Input: part model. Units: mm. Frame: model coordinates. Give positions to 0.01 mm unless a question says otherwise; leave off trailing zeros. Write each loop counter-clockwise with the first axis right and the second up, starting at its lowest first coordinate (ties: lowest second). Pieces come first, ordered by that corner, then holes. Notation, with made-up numbers: (-19.5, 11) - (33.5, 11) arc R19 cw to (33.5, 35) - close; hole circle Ø10 at (75.5, 37.5). An arc over 180 degrees is marked (long way). Use a Markdown table: item, result. Add a question column.
1. Section query C-C, the plane x = 3.55. Return loops of the section in (y, z), plus the area to 3 significant figures.
2. Section query D-D, the plane z = -0.25. Return loops of the section in (x, y), plus the area to 3 significant figures.
3. Section query B-B, the plane z = 5. Return loops of the section in (x, y), plus the area to 3 significant figures.
4. Mould query, pull axis Z, two halves, no side actions, for faces 1 (the cylindrical face through (1.87, 1.58, 5.76)), 2 (the flat face through (3, 2, -7.46)), 3 (the flat face through (4, 3.2, 0)). Classes: released by +Z, released by -Z, zero draft, split by the parting line, or undercut.
5. Material intervals for probe 1 along Z at (x, y) = (2.8, 2); probe 2 along X at (y, z) = (1.75, 5); probe 3 along Z at (x, y) = (3.2, 0.45), sorted ascending.
6. Section query A-A, the plane y = 2.5. Return loops of the section in (x, z).
```python
from build123d import *

# Parameters (mm, degrees)
SKETCH1_W           = 5.409
SKETCH1_H           = 3.2004
BOSS_EXTRUDE1_DEPTH = 7.459999939
SKETCH3_R           = 1.1303
CUT_EXTRUDE1_DEPTH  = 3.2004
FILLET1_R           = 0.762


with BuildPart() as part:
    # Sketch1 → Boss-Extrude1 (new body, symmetric)
    with BuildSketch(Plane.XY):
        with Locations((2.7045, 1.6002)):
            Rectangle(SKETCH1_W, SKETCH1_H)
    extrude(amount=BOSS_EXTRUDE1_DEPTH, both=True)

    # Sketch3 → Cut-Extrude1 (cut)
    with BuildSketch(Plane.XZ):
        with Locations((2.7045, 4.999999969)):
            Circle(SKETCH3_R)
        with Locations((2.7045, -4.999999969)):
            Circle(SKETCH3_R)
        with Locations((2.7045, 0)):
            Circle(SKETCH3_R)
    extrude(amount=-CUT_EXTRUDE1_DEPTH, mode=Mode.SUBTRACT)

    # Fillet1
    fillet1_edges = [part.edges().sort_by_distance(p)[0] for p in [
        (5.409, 1.6002, 7.459999939),
        (5.409, 1.6002, -7.459999939),
        (0, 1.6002, -7.459999939),
        (0, 1.6002, 7.459999939),
    ]]
    fillet(fillet1_edges, radius=FILLET1_R)


solid = part.part
```
Result sheet:
| question | item | result |
|---|---|---|
| 1 | outline | (0, -7.46) - (3.2, -7.46) - (3.2, -5.75) - (0, -5.75) - close; (0, -4.25) - (3.2, -4.25) - (3.2, -0.75) - (0, -0.75) - close; (0, 0.75) - (3.2, 0.75) - (3.2, 4.25) - (0, 4.25) - close; (0, 5.75) - (3.2, 5.75) - (3.2, 7.46) - (0, 7.46) - close |
| 1 | area | 33.3 mm² |
| 2 | outline | (0, 0) - (1.6, 0) - (1.6, 3.2) - (0, 3.2) - close; (3.81, 0) - (5.41, 0) - (5.41, 3.2) - (3.81, 3.2) - close |
| 2 | area | 10.3 mm² |
| 3 | outline | (0, 0) - (1.57, 0) - (1.57, 3.2) - (0, 3.2) - close; (3.83, 0) - (5.41, 0) - (5.41, 3.2) - (3.83, 3.2) - close |
| 3 | area | 10.1 mm² |
| 4 | face 1 | undercut |
| 4 | face 2 | released by -Z |
| 4 | face 3 | zero draft |
| 5 | probe 1 | z = -7.46 to -6.13, -3.87 to -1.13, 1.13 to 3.87, 6.13 to 7.46 |
| 5 | probe 2 | x = 0 to 1.57, 3.83 to 5.41 |
| 5 | probe 3 | z = -7.46 to -6.02, -3.98 to -1.02, 1.02 to 3.98, 6.02 to 7.46 |
| 6 | outline | (0, -6.7) arc R0.76 ccw to (0.76, -7.46) - (4.65, -7.46) arc R0.76 ccw to (5.41, -6.7) - (5.41, 6.7) arc R0.76 ccw to (4.65, 7.46) - (0.76, 7.46) arc R0.76 ccw to (0, 6.7) - close; hole circle Ø2.26 at (2.7, -5); hole circle Ø2.26 at (2.7, 0); hole circle Ø2.26 at (2.7, 5) |
